```python
from build123d import *

# Parameters (mm, degrees)
SKETCH1_R           = 31.525
BOSS_EXTRUDE1_DEPTH = 100
SKETCH3_R           = 30.025
CUT_EXTRUDE1_DEPTH  = 95
CHAMFER2_SIZE       = 5


with BuildPart() as part:
    # Sketch1 → Boss-Extrude1 (new body)
    with BuildSketch(Plane(origin=(0, 0, 0), x_dir=(0, 0, -1), z_dir=(1, 0, 0))):
        with Locations(Location((0, 0, 0), (0, 0, 180))):
            Circle(SKETCH1_R)
    extrude(amount=BOSS_EXTRUDE1_DEPTH)

    # Sketch3 → Cut-Extrude1 (cut)
    with BuildSketch(Plane(origin=(100, 0, 0), x_dir=(0, 0, -1), z_dir=(1, 0, 0))):
        Circle(SKETCH3_R)
    extrude(amount=-CUT_EXTRUDE1_DEPTH, mode=Mode.SUBTRACT)

    # Chamfer2
    chamfer2_edges = [part.edges().sort_by_distance(p)[0] for p in [
        (0, 0, -31.525),
    ]]
    chamfer(chamfer2_edges, length=CHAMFER2_SIZE)


solid = part.part
```
Part model, mm, in its own coordinate system. A direction names the side the tool comes from. Give positions to 0.01 mm unless a question says otherwise; leave off trailing zeros. Write each loop counter-clockwise with the first axis right and the second up, starting at its lowest first coordinate (ties: lowest second). Pieces come first, ordered by that corner, then holes. Notation, with made-up numbers: M 53.25,-10.5 L 103.25,-10.5 A26 ccw 103.25,8.5 Z; hole C 53.5,27.5 d9. An arc over 180 degrees is marked long. Use CSV: the item, a comma, the result in double quotes.
Item 1: Slice it at A-A on y = 0. Write the cut outline in (x, z) (3 decimals), plus the area to 3 significant figures.
Taken from the geometry:
outline,"M 0,-26.525 L 5,-31.525 L 100,-31.525 L 100,-30.025 L 5,-30.025 L 5,30.025 L 100,30.025 L 100,31.525 L 5,31.525 L 0,26.525 Z"
area,"575 mm²"
Item 2: Drill centre lines: probe 1 along Y at (x, z) = (38.5, 0) (3 decimals); probe 2 along X at (y, z) = (12, 17.5); probe 3 along Z at (x, y) = (17, 18). Where is each one in solid material? Low to high.
Taken from the geometry:
probe 1,"y = -31.525 to -30.025, 30.025 to 31.525"
probe 2,"x = 0 to 5"
probe 3,"z = -25.88 to -24.03, 24.03 to 25.88"
Item 3: Slice it at B-B on x = 45. Write the cut outline in (y, z) (3 decimals), plus the area to 3 significant figures.
Taken from the geometry:
outline,"C 0,0 d63.05; hole C 0,0 d60.05"
area,"290 mm²"
Item 4: Pin check, flat tips, straight feed: P1, Ø12, axis at x = 82, z = 0.5, coming from the +Y side (3 decimals); P2, Ø5, axis at x = 68, y = 6, coming from the -Z side; P3, Ø18, axis at y = -13.5, z = -12.5, coming from the +X side. Stop position of each tip, or through.
Taken from the geometry:
P1,"stops at y = 31.525"
P2,"stops at z = -31.33"
P3,"stops at x = 5"
Item 5: Pull direction Y, two halves, no side cores. Call faces 3 (the face through (53.16, -29.31, 6.51)), 4 (the face through (0.24, 26.13, -5.8)), 5 (the face through (0, 0, 0)): +Y half, -Y half, draft (parallel to the pull), parting line (faces both ways), or undercut.
Taken from the geometry:
face 3,"undercut"
face 4,"parting line"
face 5,"draft"
Item 6: Which spindle directions (+Z, -Z, +X, -X, +Y, -Y) get a long thin tool onto all of the face, cutting with end or side? Do faces 1 (the face through (51.835, 30.775, -6.834)), 2 (the face through (5, 0, 0)). Say none if no direction does.
Taken from the geometry:
face 1,"+X, -X"
face 2,"+X"
